Could you check a few things on this model? Use its own coordinates, in mm. A direction names the side the tool comes from. Round coordinates to 2 decimals unless told otherwise and drop trailing zeros. Loops run counter-clockwise (first coordinate to the right, second up) from the corner with the lowest first, then second, coordinate; pieces in that order, holes last.
Autodesk Inventor part; units mm, degrees
ref_plane "YZ Plane" through (0, 0, 0) normal (1, 0, 0) x (0, 1, 0)
ref_plane "XZ Plane" through (0, 0, 0) normal (0, 1, 0) x (-1, 0, 0)
ref_plane "XY Plane" through (0, 0, 0) normal (0, 0, 1) x (1, 0, 0)
sketch "Sketch1" plane through (0, 0, 0) normal (0, 0, 1) x (1, 0, 0)
  circle A0 centre (0, 0) radius 44.45
  dimension "d0" = 88.9
extrude "Extrusion1" add sketch "Sketch1" against normal blind 6.35
sketch "Sketch2" plane through (0, 0, 0) normal (0, 0, 1) x (1, 0, 0)
  circle A0 centre (0, 0) radius 44.45 construction
  circle A1 centre (0, 0) radius 38.1 construction
  point P0 (0, 38.1)
  dimension "d3" = 76.2
hole "Hole1" at (0, 38.1, 0) direction (0, 0, -1) diameter 5.1054 end through all
pattern_circular "Circular Pattern1" count 8 over 360 about axis through (0, 0, 0) along (0, 0, -1) of "Hole1"
sketch "Sketch3" plane through (0, 0, 0) normal (0, 0, 1) x (1, 0, 0)
  circle A0 centre (0, 0) radius 26.1938
  dimension "d14" = 52.3875
extrude "Extrusion2" cut sketch "Sketch3" against normal blind 1.5875
properties part number "EL2-A-003" material "Aluminum 6061"
Item 1: For faces 1 (the cylindrical face through (-28.97, 25.39, -3.22)), 2 (the flat face through (0, 0, -1.588)), which set-ups out of +Z, -Z, +X, -X, +Y, -Y let a thin tool reach every point of the face, with its end or its side?
Results list:
face 1: +Z, -Z
face 2: +Z
Item 2: If we section it at A-A, the plane y = 0: Please give me the cut outline in (x, z).
Results list:
outline: (-44.45, -6.35) - (-40.65, -6.35) - (-40.65, 0) - (-44.45, 0) - close; (-35.55, -6.35) - (35.55, -6.35) - (35.55, 0) - (26.19, 0) - (26.19, -1.59) - (-26.19, -1.59) - (-26.19, 0) - (-35.55, 0) - close; (40.65, -6.35) - (44.45, -6.35) - (44.45, 0) - (40.65, 0) - close
Item 3: If we section it at D-D, the plane z = -3: Count the separate pieces of the cut face and the enclosed holes in it, then the cut area to 3 significant figures.
Results list:
separate pieces: 1
enclosed holes: 8
area: 6,040 mm2
Item 4: Will these pins go through, and if not, where does the flat tip stop? pin 1 (1 mm diameter, centred on x = 19.5, y = -29.5, fed in from +Z); pin 2 (4 mm diameter, centred on x = 26.94, y = 26.94, fed in from -Z); pin 3 (2 mm diameter, centred on y = -3.5, z = -2.5, fed in from +X); pin 4 (3 mm diameter, centred on x = -24.5, z = -4, fed in from -Y).
Results list:
pin 1: stops at z = 0
pin 2: passes through
pin 3: stops at x = 44.38
pin 4: stops at y = -38.04
Item 5: If I drill on line 1 along Y through (x, z) = (27, -0.5); line 2 along X through (y, z) = (-27.5, -1.5); line 3 along Z through (x, y) = (10, 20), over which ranges is the centre line in solid material (lowest first)?
Results list:
line 1: y = -35.31 to -29.49, -24.39 to 24.39, 29.49 to 35.31
line 2: x = -34.92 to -29.43, -24.45 to 24.45, 29.43 to 34.92
line 3: z = -6.35 to -1.59
Item 6: If we section it at C-C, the plane x = -38.1: Please give me the cut outline in (y, z).
Results list:
outline: (-22.9, -6.35) - (-2.55, -6.35) - (-2.55, 0) - (-22.9, 0) - close; (2.55, -6.35) - (22.9, -6.35) - (22.9, 0) - (2.55, 0) - close
